For this review, use the dimensioned drawing (mm, ordinates from the lowest corner) and the shaded views. Round coordinates to 2 decimals unless told otherwise and drop trailing zeros. Use CSV: the item, a comma, the result in double quotes.
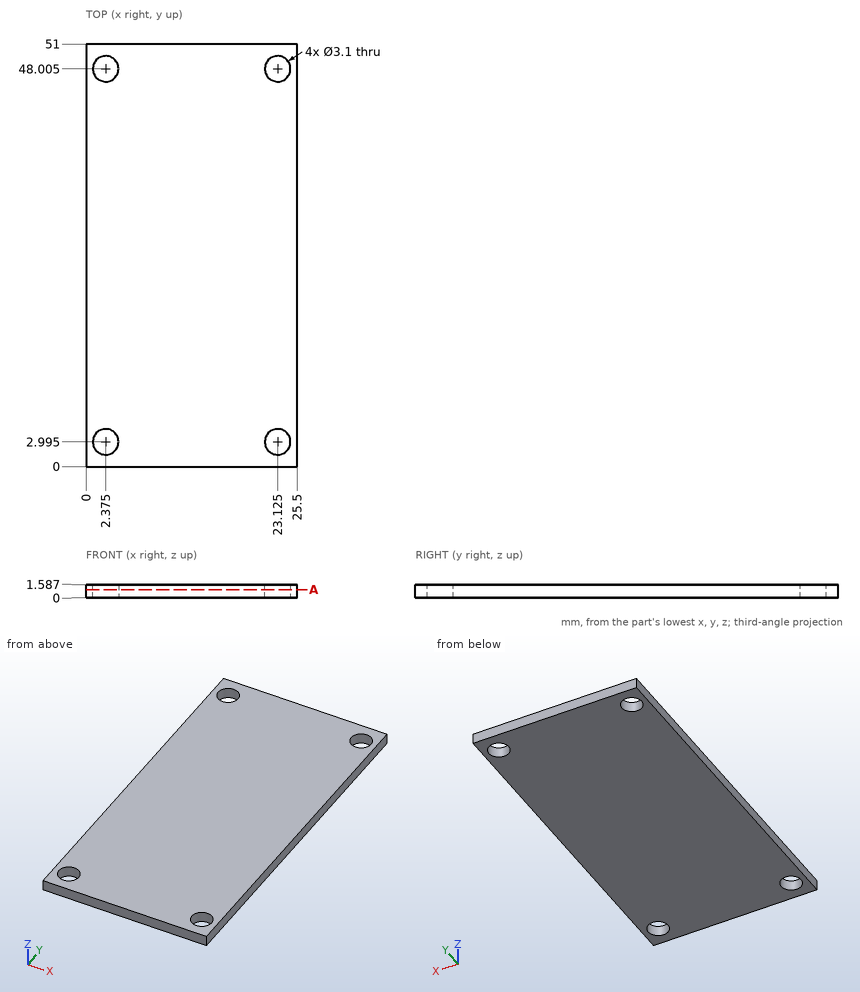
1) Wall thickness on line 1 along Y through (x, z) = (23, 0.45); line 2 along X through (y, z) = (48, 1.35) (1 decimal); line 3 along Y through (x, z) = (22, 0.35): over which ranges is each line inside the solid? List them lowest first. Write a range as [from, to].
Answers:
line 1,"[0, 1.45], [4.54, 46.46], [49.55, 51]"
line 2,"[0, 0.8], [3.9, 21.6], [24.7, 25.5]"
line 3,"[0, 1.93], [4.06, 46.94], [49.07, 51]"
2) Add section A-A on z = 1. Give the number of separate pieces and of enclosed holes in the cut face, then the cut area to 3 significant figures.
Answers:
separate pieces,"1"
enclosed holes,"4"
area,"1,270 mm²"
3) For pin 1 Ø1.9 at (x, y) = (23.125, 48.005) entering from -Z, flat-tipped, find the tip position at first contact; note if it passes through.
Answers:
pin 1,"through"
